Geometry: see drawing. Coordinates: mm, zero at the bounding-box minimum. Give positions to 0.01 mm unless a question says otherwise; leave off trailing zeros. Loops run counter-clockwise (first coordinate to the right, second up) from the corner with the lowest first, then second, coordinate; pieces in that order, holes last. Notation, with made-up numbers: (78.25, 74.25) -> (83.25, 74.25) arc R22 ccw to (83.25, 81.25) -> close; hole circle Ø7 at (-11, 87). An arc over 180 degrees is marked (long way). Return JSON: item names as keys, results as strings. Group by question number.
(1) Ray query, line 1 (X direction, y = 25, z = 0.9) (1 decimal); line 2 (X direction, y = 10.5, z = 2.55); line 3 (Y direction, x = 71.5, z = 1.7). Return the intervals inside material, ascending. Write a range as from..to.
(2) Pin query (flat end, axial travel): pin 1 (4 mm diameter, centred on x = 17.17, y = 124.9, fed in from +Z); pin 2 (1.5 mm diameter, centred on y = 5, z = 1, fed in from +X); pin 3 (1.5 mm diameter, centred on y = 11.5, z = 1.5, fed in from -X); pin 4 (0.9 mm diameter, centred on x = 70.5, z = 1, fed in from -Y). Return the tip coordinate at first contact, or that it passes through.
(3) Cut plane B-B on x = 46.5. Return loops of the section in (y, z).
(4) Cut plane C-C on y = 36.5. Return loops of the section in (x, z).
(5) Cut plane A-A on z = 2.35. Give the number of separate pieces and of enclosed holes in the cut face, then the cut area to 3 significant figures.
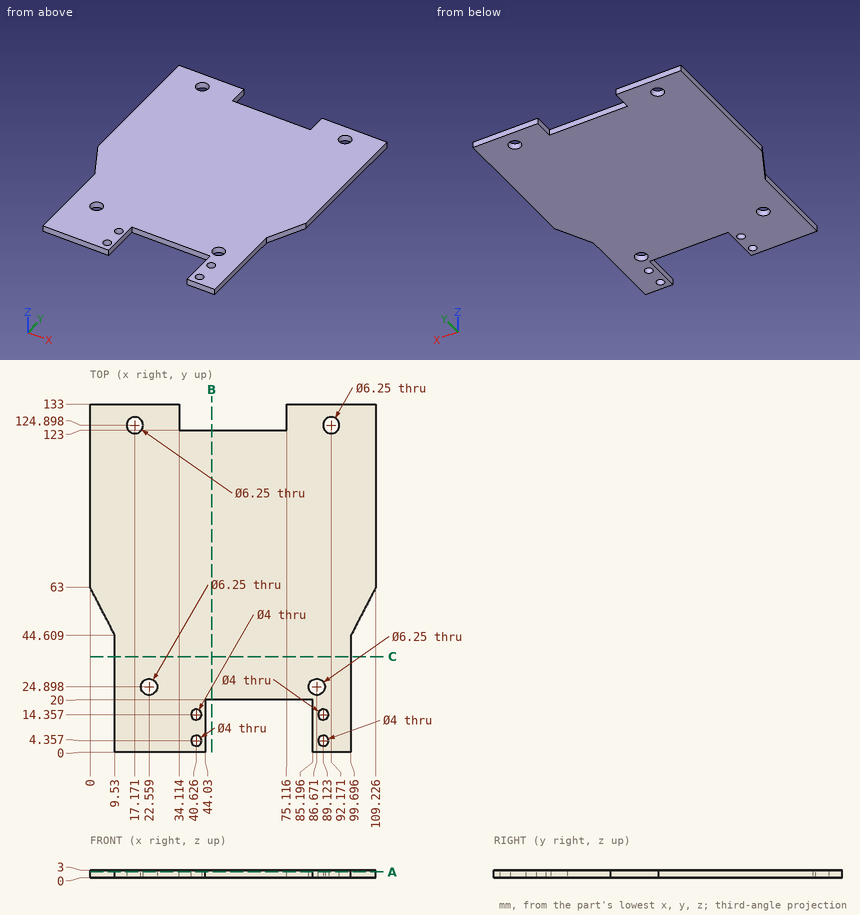
Answers:
{
 "1": {"line 1": "9.5..19.4, 25.7..83.5, 89.8..99.7", "line 2": "9.53..44.03, 85.2..99.7", "line 3": "20..123"},
 "2": {"pin 1": "through", "pin 2": "x = 99.7", "pin 3": "x = 9.53", "pin 4": "y = 20"},
 "3": {"outline": "(20, 0) -> (123, 0) -> (123, 3) -> (20, 3) -> close"},
 "4": {"outline": "(9.53, 0) -> (99.7, 0) -> (99.7, 3) -> (9.53, 3) -> close"},
 "5": {"separate pieces": "1", "enclosed holes": "8", "area": "12,100 mm²"}
}
